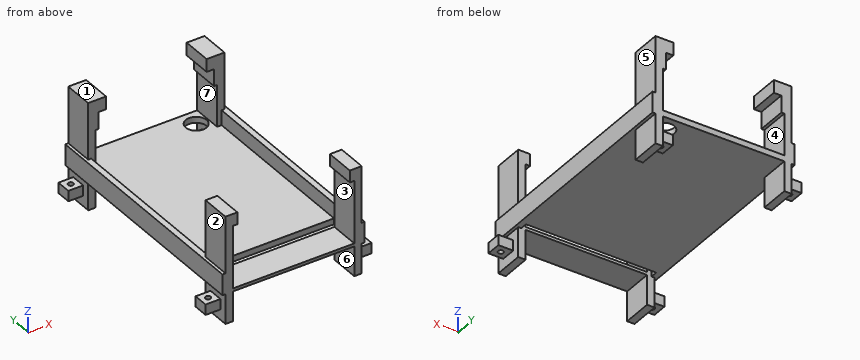
from build123d import *

# Parameters (mm, degrees)
CYLINDER013_R     = 3.5
CYLINDER013_DEPTH = 15
CYLINDER012_R     = 0.9
CYLINDER012_DEPTH = 3.5
BOX039_W          = 5
BOX039_H          = 5
BOX039_DEPTH      = 3.5
BOX036_W          = 2.5
BOX036_H          = 10
BOX036_DEPTH      = 36
BOX031_W          = 1
BOX031_H          = 10
BOX031_DEPTH      = 10
BOX029_W          = 1.5
BOX029_H          = 10
BOX029_DEPTH      = 4
BOX032_W          = 2.5
BOX032_H          = 10
BOX032_DEPTH      = 4.3
BOX037_W          = 2
BOX037_H          = 78.9
BOX037_DEPTH      = 7
BOX033_W          = 2
BOX033_H          = 78.9
BOX033_DEPTH      = 7
BOX030_W          = 2.5
BOX030_H          = 10
BOX030_DEPTH      = 36
BOX034_W          = 45.8
BOX034_H          = 66.5
BOX034_DEPTH      = 2
BOX038_W          = 45.8
BOX038_H          = 10
BOX038_DEPTH      = 1
BOX035_W          = 2.5
BOX035_H          = 10
BOX035_DEPTH      = 36
BOX028_W          = 2.5
BOX028_H          = 10
BOX028_DEPTH      = 36


with BuildPart() as anchorhole003:
    # Cylinder013 → Cylinder013 (new body)
    with BuildSketch(Plane(origin=(2.5, 2.5, 0), x_dir=(1, 0, 0), z_dir=(0, 0, 1))):
        Circle(CYLINDER013_R)
    extrude(amount=CYLINDER013_DEPTH)


with BuildPart() as anchorhole003_1:
    # Clone024 placement: moved
    add(anchorhole003.part.moved(Location((76.9, 78, 9))))


with BuildPart() as anchorscrew:
    # Cylinder012 → Cylinder012 (new body)
    with BuildSketch(Plane(origin=(2.5, 2.5, 0), x_dir=(1, 0, 0), z_dir=(0, 0, 1))):
        Circle(CYLINDER012_R)
    extrude(amount=CYLINDER012_DEPTH)


with BuildPart() as anchor:
    # Box039 → Box039 (new body)
    with BuildSketch(Plane.XY):
        with Locations((2.5, 2.5)):
            Rectangle(BOX039_W, BOX039_H)
    extrude(amount=BOX039_DEPTH)

    # Cut010: cut AnchorScrew
    add(anchorscrew.part, mode=Mode.SUBTRACT)


with BuildPart() as anchor001:
    # Clone005 base: copy of Anchor
    add(anchor.part)


with BuildPart() as anchor001_1:
    # Clone005 placement: moved
    add(anchor001.part.moved(Location((85.9, 9.6, 2))))


with BuildPart() as part_mirroring004:
    # Part__Mirroring004: instance of anchor001
    add(anchor001_1.part.mirror(Plane(origin=(0, 0, 5.5), x_dir=(0, 1, 0), z_dir=(0, 0, 1))))


with BuildPart() as clone006:
    # Clone006 base: copy of Anchor
    add(anchor.part)


with BuildPart() as clone006_1:
    # Clone006 placement: moved
    add(clone006.part.moved(Location((78.4, 78.5, 2))))


with BuildPart() as part_mirroring005:
    # Part__Mirroring005: instance of Clone006
    add(clone006_1.part.mirror(Plane(origin=(0, 0, 5.5), x_dir=(0, 1, 0), z_dir=(0, 0, 1))))


with BuildPart() as cube028:
    # Box036 → Box036 (new body)
    with BuildSketch(Plane(origin=(83.4, 76, 2), x_dir=(1, 0, 0), z_dir=(0, 0, 1))):
        with Locations((1.25, 5)):
            Rectangle(BOX036_W, BOX036_H)
    extrude(amount=BOX036_DEPTH)


with BuildPart() as cube023:
    # Box031 → Box031 (new body)
    with BuildSketch(Plane(origin=(42.6, 76, 28), x_dir=(1, 0, 0), z_dir=(0, 0, 1))):
        with Locations((0.5, 5)):
            Rectangle(BOX031_W, BOX031_H)
    extrude(amount=BOX031_DEPTH)


with BuildPart() as cube021:
    # Box029 → Box029 (new body)
    with BuildSketch(Plane(origin=(42.6, 7.1, 34), x_dir=(1, 0, 0), z_dir=(0, 0, 1))):
        with Locations((0.75, 5)):
            Rectangle(BOX029_W, BOX029_H)
    extrude(amount=BOX029_DEPTH)


with BuildPart() as fusion004:
    # Box032 → Box032 (new body)
    with BuildSketch(Plane(origin=(43.6, 76, 33.7), x_dir=(1, 0, 0), z_dir=(0, 0, 1))):
        with Locations((1.25, 5)):
            Rectangle(BOX032_W, BOX032_H)
    extrude(amount=BOX032_DEPTH)

    # Fusion004: union Cube023, Cube021
    add(cube023.part)
    add(cube021.part)


with BuildPart() as part_mirroring003:
    # Part__Mirroring003: instance of Fusion004
    add(fusion004.part.mirror(Plane(origin=(63, 0, 0), x_dir=(0, -1, 0), z_dir=(1, 0, 0))))


with BuildPart() as anchor003:
    # Clone008 base: copy of Anchor
    add(anchor.part)


with BuildPart() as anchor003_1:
    # Clone008 placement: moved
    add(anchor003.part.moved(Location((35.1, 78.5, 2))))


with BuildPart() as part_mirroring007:
    # Part__Mirroring007: instance of Anchor003
    add(anchor003_1.part.mirror(Plane(origin=(0, 0, 5.5), x_dir=(0, 1, 0), z_dir=(0, 0, 1))))


with BuildPart() as cube029:
    # Box037 → Box037 (new body)
    with BuildSketch(Plane(origin=(84.9, 7.1, 12), x_dir=(1, 0, 0), z_dir=(0, 0, 1))):
        with Locations((1, 39.45)):
            Rectangle(BOX037_W, BOX037_H)
    extrude(amount=BOX037_DEPTH)


with BuildPart() as cube025:
    # Box033 → Box033 (new body)
    with BuildSketch(Plane(origin=(39.1, 7.1, 12), x_dir=(1, 0, 0), z_dir=(0, 0, 1))):
        with Locations((1, 39.45)):
            Rectangle(BOX033_W, BOX033_H)
    extrude(amount=BOX033_DEPTH)


with BuildPart() as cube022:
    # Box030 → Box030 (new body)
    with BuildSketch(Plane(origin=(40.1, 76, 2), x_dir=(1, 0, 0), z_dir=(0, 0, 1))):
        with Locations((1.25, 5)):
            Rectangle(BOX030_W, BOX030_H)
    extrude(amount=BOX030_DEPTH)


with BuildPart() as cube026:
    # Box034 → Box034 (new body)
    with BuildSketch(Plane(origin=(40.1, 19.5, 12), x_dir=(1, 0, 0), z_dir=(0, 0, 1))):
        with Locations((22.9, 33.25)):
            Rectangle(BOX034_W, BOX034_H)
    extrude(amount=BOX034_DEPTH)


with BuildPart() as anchor002:
    # Clone007 base: copy of Anchor
    add(anchor.part)


with BuildPart() as anchor002_1:
    # Clone007 placement: moved
    add(anchor002.part.moved(Location((35.1, 9.6, 2))))


with BuildPart() as part_mirroring006:
    # Part__Mirroring006: instance of Anchor002
    add(anchor002_1.part.mirror(Plane(origin=(0, 0, 5.5), x_dir=(0, 1, 0), z_dir=(0, 0, 1))))


with BuildPart() as cube030:
    # Box038 → Box038 (new body)
    with BuildSketch(Plane(origin=(40.1, 7.1, 12), x_dir=(1, 0, 0), z_dir=(0, 0, 1))):
        with Locations((22.9, 5)):
            Rectangle(BOX038_W, BOX038_H)
    extrude(amount=BOX038_DEPTH)


with BuildPart() as cube027:
    # Box035 → Box035 (new body)
    with BuildSketch(Plane(origin=(83.4, 7.1, 2), x_dir=(1, 0, 0), z_dir=(0, 0, 1))):
        with Locations((1.25, 5)):
            Rectangle(BOX035_W, BOX035_H)
    extrude(amount=BOX035_DEPTH)


with BuildPart() as flashercradle:
    # Box028 → Box028 (new body)
    with BuildSketch(Plane(origin=(40.1, 7.1, 2), x_dir=(1, 0, 0), z_dir=(0, 0, 1))):
        with Locations((1.25, 5)):
            Rectangle(BOX028_W, BOX028_H)
    extrude(amount=BOX028_DEPTH)

    # Fusion005: union Part__Mirroring004, Part__Mirroring005, Cube028, Part__Mirroring003, Part__Mirroring007, Cube029, Cube025, Cube022, Cube026, Part__Mirroring006, Cube030, Cube027, Fusion004
    add(part_mirroring004.part)
    add(part_mirroring005.part)
    add(cube028.part)
    add(part_mirroring003.part)
    add(part_mirroring007.part)
    add(cube029.part)
    add(cube025.part)
    add(cube022.part)
    add(cube026.part)
    add(part_mirroring006.part)
    add(cube030.part)
    add(cube027.part)
    add(fusion004.part)

    # Cut021: cut AnchorHole003
    add(anchorhole003_1.part, mode=Mode.SUBTRACT)


solid = flashercradle.part
Check sheet for the modelled part. Datum: model origin and axes. Units: mm. Face numbers are marked on the shaded views. A direction names the side the tool comes from. Round coordinates to 2 decimals unless told otherwise and drop trailing zeros. Loops run counter-clockwise (first coordinate to the right, second up) from the corner with the lowest first, then second, coordinate; pieces in that order, holes last. Notation, with made-up numbers: M 38,10 L 79,10 A23 cw 79,36 Z; hole C -30,10.5 d10. An arc over 180 degrees is marked long. One line per question, with ' | ' between items. Start each with the question number.
Item 1: Set-up check for the marked faces 5, 6 and 7: record each of +Z, -Z, +X, -X, +Y, -Y from which the full face is reachable in a straight line by a thin tool's end or side.
Item 2: Release check for a two-part mould opening along Z. For the marked faces 1, 2, 3 and 4 record: released by +Z, released by -Z, zero draft, split by the parting line, or undercut.
Item 3: Section check D-D (z = 17). Record the boundary of the cut face in (x, y), and give its area (3 significant figures).
Item 4: Section check A-A (x = 88.4). Record the boundary of the cut face in (y, z), and give its area (3 significant figures).
Item 5: Section check B-B (z = 25.5). Record the boundary of the cut face in (x, y), and give its area (3 significant figures).
Item 6: Section check C-C (y = 27). Record the boundary of the cut face in (x, z).
Item 7: Scan lines: probe 1 along X at (y, z) = (12, 7); probe 2 along Y at (x, z) = (79.4, 12.7); probe 3 along Z at (x, y) = (44.5, 80.5). Record each from-to range of solid material in increasing order.
Item 8: Gauge pin test, flat ends, axial feed: pin 1 Ø8 at (y, z) = (79, 30) entering from +X; pin 2 Ø3 at (x, z) = (81, 7) entering from -Y; pin 3 Ø5 at (y, z) = (57.5, 10.5) entering from +X. Record the tip position at first contact, or that the pin passes through.
Worked out:
1) face 5: +Z, +X, +Y, -Y | face 6: -Z, -Y | face 7: +Y, -Y
2) face 1: released by +Z | face 2: zero draft | face 3: undercut | face 4: undercut
3) outline: M 39.1,7.1 L 42.6,7.1 L 42.6,17.1 L 41.1,17.1 L 41.1,76 L 42.6,76 L 42.6,86 L 39.1,86 Z; M 83.4,7.1 L 86.9,7.1 L 86.9,86 L 83.4,86 L 83.4,76 L 84.9,76 L 84.9,17.1 L 83.4,17.1 Z | area: 376 mm^2
4) outline: M 9.6,5.5 L 11.2,5.5 L 11.2,9 L 9.6,9 Z; M 13,5.5 L 14.6,5.5 L 14.6,9 L 13,9 Z | area: 11.2 mm^2
5) outline: M 40.1,7.1 L 42.6,7.1 L 42.6,17.1 L 40.1,17.1 Z; M 40.1,76 L 42.6,76 L 42.6,86 L 40.1,86 Z; M 83.4,7.1 L 85.9,7.1 L 85.9,17.1 L 83.4,17.1 Z; M 83.4,76 L 85.9,76 L 85.9,86 L 83.4,86 Z | area: 100 mm^2
6) outline: M 39.1,12 L 86.9,12 L 86.9,19 L 84.9,19 L 84.9,14 L 41.1,14 L 41.1,19 L 39.1,19 Z
7) probe 1: 35.1 to 36.71, 38.49 to 42.6, 83.4 to 87.51, 89.29 to 90.9 | probe 2: 7.1 to 17.1, 19.5 to 77, 84 to 86 | probe 3: 12 to 14, 33.7 to 38
8) pin 1: x = 85.9 | pin 2: y = 78.5 | pin 3: x = 86.9
